from build123d import *

# Parameters (mm, degrees)
F0_W     = 68.3
F0_H     = 50
F0_R     = 2
F0_R_2   = 11
F1_DEPTH = 15
F2_R     = 4.25
F3_DEPTH = 50


with BuildPart() as f1:
    # F0 (on Top) → F1 (new body)
    with BuildSketch(Plane.XY):
        Rectangle(F0_W, F0_H)
        with Locations((-15.5, -15.5)):
            Circle(F0_R, mode=Mode.SUBTRACT)
        with Locations((15.5, -15.5)):
            Circle(F0_R, mode=Mode.SUBTRACT)
        with Locations((-15.5, 15.5)):
            Circle(F0_R, mode=Mode.SUBTRACT)
        Circle(F0_R_2, mode=Mode.SUBTRACT)
        with Locations((15.5, 15.5)):
            Circle(F0_R, mode=Mode.SUBTRACT)
    extrude(amount=F1_DEPTH)

    # F2 (on face) → F3 (cut, through all)
    with BuildSketch(Plane.XZ.offset(25)):
        with Locations((-26.15, 7.5)):
            Circle(F2_R)
        with Locations((26.15, 7.5)):
            Circle(F2_R)
    extrude(amount=-F3_DEPTH, mode=Mode.SUBTRACT)


solid = f1.part
Input: part model. Units: mm. Frame: model coordinates. Give positions to 0.01 mm unless a question says otherwise; leave off trailing zeros. Loops run counter-clockwise (first coordinate to the right, second up) from the corner with the lowest first, then second, coordinate; pieces in that order, holes last. Notation, with made-up numbers: (12.25, 58.25) - (36.25, 58.25) arc R19 ccw to (36.25, 83.25) - close; hole circle Ø3 at (11.25, 56.5). An arc over 180 degrees is marked (long way). Use CSV: the item, a comma, the result in double quotes. Start each with the question number.
Item 1: Contact query for a flat-ended pin moving along its axis: P1, Ø20, axis at x = 0, y = 0, coming from the +Z side. Output: stop coordinate, or through.
Item 2: Section C-C on x = -15.5. Return loops of the section in (y, z), then the cut area to 3 significant figures.
Item 3: Mould query, pull axis X, two halves, no side actions, for faces 1 (the cylindrical face through (-15.76, 17.483, 7.395)), 2 (the flat face through (0, 25, 7)), 3 (the flat face through (-34.15, 0, 7)). Classes: pulls with the +X half, pulls with the -X half, needs draft (parallel to the pull), parting line crosses it, or undercut.
Item 4: Section A-A on y = 15.5. Return loops of the section in (x, z).
Item 5: Line query: line 1 (Y direction, x = -15.5, z = 10); line 2 (X direction, y = -14.5, z = 3.75); line 3 (Z direction, x = -26, y = -8). Output: solid intervals per line, ascending.
Item 6: Section B-B on z = 9.5. Return loops of the section in (x, y), then the cut area to 3 significant figures.
Item 7: Section D-D on y = 0. Return loops of the section in (x, z).
Ans:
1,P1,"passes through"
2,outline,"(-25, 0) - (-17.5, 0) - (-17.5, 15) - (-25, 15) - close; (-13.5, 0) - (13.5, 0) - (13.5, 15) - (-13.5, 15) - close; (17.5, 0) - (25, 0) - (25, 15) - (17.5, 15) - close"
2,area,"630 mm2"
3,face 1,"undercut"
3,face 2,"needs draft"
3,face 3,"pulls with the -X half"
4,outline,"(-34.15, 0) - (-17.5, 0) - (-17.5, 15) - (-34.15, 15) - close; (-13.5, 0) - (13.5, 0) - (13.5, 15) - (-13.5, 15) - close; (17.5, 0) - (34.15, 0) - (34.15, 15) - (17.5, 15) - close; hole circle Ø8.5 at (-26.15, 7.5); hole circle Ø8.5 at (26.15, 7.5)"
5,line 1,"y = -25 to -17.5, -13.5 to 13.5, 17.5 to 25"
5,line 2,"x = -34.15 to -28.15, -24.15 to -17.23, -13.77 to 13.77, 17.23 to 24.15, 28.15 to 34.15"
5,line 3,"z = 0 to 3.25, 11.75 to 15"
6,outline,"(-34.15, -25) - (-29.9, -25) - (-29.9, 25) - (-34.15, 25) - close; (-22.4, -25) - (22.4, -25) - (22.4, 25) - (-22.4, 25) - close; (29.9, -25) - (34.15, -25) - (34.15, 25) - (29.9, 25) - close; hole circle Ø4 at (-15.5, -15.5); hole circle Ø4 at (-15.5, 15.5); hole circle Ø22 at (0, 0); hole circle Ø4 at (15.5, -15.5); hole circle Ø4 at (15.5, 15.5)"
6,area,"2,230 mm2"
7,outline,"(-34.15, 0) - (-11, 0) - (-11, 15) - (-34.15, 15) - close; (11, 0) - (34.15, 0) - (34.15, 15) - (11, 15) - close; hole circle Ø8.5 at (-26.15, 7.5); hole circle Ø8.5 at (26.15, 7.5)"
